from build123d import *

# Parameters (mm, degrees)
SKETCH1_W                = 30
SKETCH1_H                = 14
BOSS_EXTRUDE1_DEPTH      = 2
SKETCH1_9_OUTSIDE_W      = 38.634
SKETCH1_9_OUTSIDE_H      = 22.634
SKETCH1_9_OUTSIDE_W_2    = 30
SKETCH1_9_OUTSIDE_H_2    = 14
SKETCH1_9_OUTSIDE_R      = 2
CUT_EXTRUDE10_DEPTH      = 3
CUT_EXTRUDE10_DEPTH_BACK = 1


with BuildPart() as part:
    # Sketch1 → Boss-Extrude1 (new body)
    with BuildSketch(Plane(origin=(0, 0, 0), x_dir=(1, 0, 0), z_dir=(0, 1, 0))):
        with Locations((-15, 7)):
            Rectangle(SKETCH1_W, SKETCH1_H)
    extrude(amount=BOSS_EXTRUDE1_DEPTH)

    # Sketch1<9> outside → Cut-Extrude10 (cut, two sides)
    with BuildSketch(Plane(origin=(0, 0, 0), x_dir=(1, 0, 0), z_dir=(0, 1, 0))) as cut_extrude10_sk:
        with Locations((-15, 7)):
            Rectangle(SKETCH1_9_OUTSIDE_W, SKETCH1_9_OUTSIDE_H)
        with Locations((-15, 7)):
            Rectangle(SKETCH1_9_OUTSIDE_W_2, SKETCH1_9_OUTSIDE_H_2, mode=Mode.SUBTRACT)
        with Locations((-7.020370045, 7)):
            Circle(SKETCH1_9_OUTSIDE_R)
    extrude(amount=CUT_EXTRUDE10_DEPTH, mode=Mode.SUBTRACT)
    extrude(cut_extrude10_sk.sketch, amount=-CUT_EXTRUDE10_DEPTH_BACK, mode=Mode.SUBTRACT)


solid = part.part
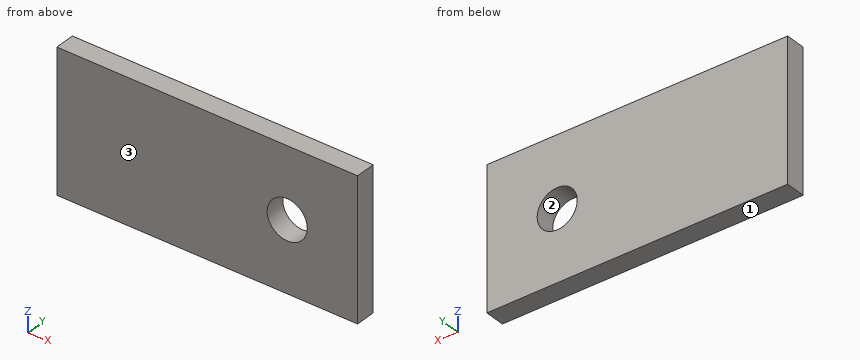
Input: part model. Units: mm. Frame: model coordinates. Face numbers are marked on the shaded views. Give positions to 0.01 mm unless a question says otherwise; leave off trailing zeros. Loops run counter-clockwise (first coordinate to the right, second up) from the corner with the lowest first, then second, coordinate; pieces in that order, holes last. Notation, with made-up numbers: (-38, -11) -> (-10, -11) arc R21 cw to (-10, 26) -> close; hole circle Ø4 at (33.25, -30.75). An arc over 180 degrees is marked (long way). Answer as a JSON object with one key per item and string values. Group by question number.
Item 1: Line query: probe 1 along X at (y, z) = (0.75, -7); probe 2 along X at (y, z) = (1.35, -7.75). Output: solid intervals per line, ascending.
Item 2: Cut plane C-C, the plane z = -5.5. Return the cut outline in (x, y).
Item 3: Pull-direction query (Z, two-part tool) for the marked faces 1, 2 and 3; classes: released by +Z, released by -Z, zero draft, split by the parting line, or undercut.
Item 4: Cut plane A-A, the plane z = -7. Return the cut outline in (x, y).
Item 5: Pin query (flat end, axial travel): P1, Ø2.5, axis at x = -7.02, z = -7, coming from the +Y side. Return the tip coordinate at first contact, or that it passes through.
Item 6: Cut plane B-B, the plane y = 0.7. Return the cut outline in (x, z), and give its area (3 significant figures).
Checks:
{
 "1": {"probe 1": "x = -30 to -9.02, -5.02 to 0", "probe 2": "x = -30 to -8.87, -5.17 to 0"},
 "2": {"outline": "(-30, 0) -> (-8.34, 0) -> (-8.34, 2) -> (-30, 2) -> close; (-5.7, 0) -> (0, 0) -> (0, 2) -> (-5.7, 2) -> close"},
 "3": {"face 1": "released by -Z", "face 2": "undercut", "face 3": "zero draft"},
 "4": {"outline": "(-30, 0) -> (-9.02, 0) -> (-9.02, 2) -> (-30, 2) -> close; (-5.02, 0) -> (0, 0) -> (0, 2) -> (-5.02, 2) -> close"},
 "5": {"P1": "passes through"},
 "6": {"outline": "(-30, -14) -> (0, -14) -> (0, 0) -> (-30, 0) -> close; hole circle Ø4 at (-7.02, -7)", "area": "407 mm²"}
}
